Can you work these out from the model? Positions are in its coordinate system, mm. A direction names the side the tool comes from. Coordinates: 2 decimals unless noted, no trailing zeros. Loops run counter-clockwise (first coordinate to the right, second up) from the corner with the lowest first, then second, coordinate; pieces in that order, holes last.
```python
from build123d import *

# Parameters (mm, degrees)
SKETCH2_R           = 1.75
BOSS_EXTRUDE1_DEPTH = 5
FILLET1_R           = 5
SKETCH3_R           = 3.5
SKETCH3_W           = 2.1
SKETCH3_H           = 10.1
CUT_EXTRUDE1_DEPTH  = 6


with BuildPart() as part:
    # Sketch2 → Boss-Extrude1 (new body)
    with BuildSketch(Plane(origin=(0, 0, 0), x_dir=(1, 0, 0), z_dir=(0, 1, 0))):
        with BuildLine():
            Line((3, 28.141242251), (3, 32.361242251))
            ThreePointArc((3, 32.361242251), (0, 32.5), (-3, 32.361242251))
            Line((-3, 32.361242251), (-3, 28.141242251))
            Line((-3, 28.141242251), (-11.25, 28.141242251))
            Line((-11.25, 28.141242251), (-11.25, 22.141242251))
            Line((-11.25, 22.141242251), (-20.976543843, 22.141242251))
            ThreePointArc((-20.976543843, 22.141242251), (-30.5, 0), (-20.976543843, -22.141242251))
            Line((-20.976543843, -22.141242251), (-11.25, -22.141242251))
            Line((-11.25, -22.141242251), (-11.25, -28.141242251))
            Line((-11.25, -28.141242251), (-3, -28.141242251))
            Line((-3, -28.141242251), (-3, -32.361242251))
            ThreePointArc((-3, -32.361242251), (0, -32.5), (3, -32.361242251))
            Line((3, -32.361242251), (3, -28.141242251))
            Line((3, -28.141242251), (11.25, -28.141242251))
            Line((11.25, -28.141242251), (11.25, -22.141242251))
            Line((11.25, -22.141242251), (20.976543843, -22.141242251))
            ThreePointArc((20.976543843, -22.141242251), (30.5, 0), (20.976543843, 22.141242251))
            Line((20.976543843, 22.141242251), (11.25, 22.141242251))
            Line((11.25, 22.141242251), (11.25, 28.141242251))
            Line((11.25, 28.141242251), (3, 28.141242251))
        make_face()
        with Locations((0, 29.32)):
            Circle(SKETCH2_R, mode=Mode.SUBTRACT)
        with Locations((0, -29.32)):
            Circle(SKETCH2_R, mode=Mode.SUBTRACT)
    extrude(amount=BOSS_EXTRUDE1_DEPTH)

    # Fillet1
    fillet1_edges = [part.edges().sort_by_distance(p)[0] for p in [
        (-11.25, 2.5, -22.141242251),
        (11.25, 2.5, -22.141242251),
        (11.25, 2.5, 22.141242251),
        (-11.25, 2.5, 22.141242251),
    ]]
    fillet(fillet1_edges, radius=FILLET1_R)

    # Sketch3 → Cut-Extrude1 (cut, through all)
    with BuildSketch(Plane(origin=(0, 5, 0), x_dir=(1, 0, 0), z_dir=(0, 1, 0))):
        with Locations((10.253456157, 10.021242251)):
            Circle(SKETCH3_R)
        with Locations((-15.293456157, -16.411242251)):
            Circle(SKETCH3_R)
        with Locations((-20.976543843, -6.771242251)):
            Rectangle(SKETCH3_W, SKETCH3_H)
    extrude(amount=-CUT_EXTRUDE1_DEPTH, mode=Mode.SUBTRACT)


solid = part.part
```
Item 1: I need wall thicknesses on line 1 along Z through (x, y) = (0, 1.25); line 2 along Z through (x, y) = (-0.5, 1.1); line 3 along Z through (x, y) = (-5.5, 0.3). Which ranges of each line are inside material? Lowest first, please.
Results are:
line 1: z = -32.5 to -31.07, -27.57 to 27.57, 31.07 to 32.5
line 2: z = -32.5 to -31, -27.64 to 27.64, 31 to 32.5
line 3: z = -28.14 to 28.14
Item 2: Suppose I cut it at A-A, the plane z = 29.32. Please give me the cut outline in (x, y).
Results are:
outline: (-3, 0) - (-1.75, 0) - (-1.75, 5) - (-3, 5) - close; (1.75, 0) - (3, 0) - (3, 5) - (1.75, 5) - close
Item 3: Suppose I cut it at B-B, the plane x = 0. Please give me the cut outline in (y, z), plus the area to 3 significant figures.
Results are:
outline: (0, -32.5) - (5, -32.5) - (5, -31.07) - (0, -31.07) - close; (0, -27.57) - (5, -27.57) - (5, 27.57) - (0, 27.57) - close; (0, 31.07) - (5, 31.07) - (5, 32.5) - (0, 32.5) - close
area: 290 mm2
Item 4: We'd pull the mould along Z, two halves only. Please class faces 4 (the face through (-7, 2, 28.141)), 5 (the face through (-12.68, 2.54, -23.64)), 6 (the face through (13.592, 2.535, -11.073)): +Z half, -Z half, draft (parallel to the pull), parting line (faces both ways), or undercut.
Results are:
face 4: +Z half
face 5: -Z half
face 6: undercut
Item 5: Suppose I cut it at D-D, the plane z = 7. Please give me the cut outline in (x, y).
Results are:
outline: (-29.69, 0) - (-22.03, 0) - (-22.03, 5) - (-29.69, 5) - close; (-19.93, 0) - (29.69, 0) - (29.69, 5) - (-19.93, 5) - close
Item 6: I'm going to push flat-ended pins straight in: P1, Ø1.4, axis at x = 19, y = 2.5, coming from the +Z side; P2, Ø1.4, axis at x = -19, y = 3, coming from the -Z side; P3, Ø3, axis at x = -12, z = -16.5, coming from the -Y side; P4, Ø3, axis at x = 6.5, y = 4.5, coming from the +Z side. Where does each tip first touch, or does it pass through?
Results are:
P1: stops at z = 22.14
P2: stops at z = -22.14
P3: stops at y = 0
P4: stops at z = 28.14
Item 7: Suppose I cut it at C-C, the plane y = 3.45. Count the separate pieces of the cut face and the enclosed holes in it, plus the area to 3 significant figures.
Results are:
separate pieces: 1
enclosed holes: 5
area: 2,670 mm2
Item 8: On a 3-axis mill with a long thin cutter (end or side, diameter ignored), from which of +Z, -Z, +X, -X, +Y, -Y can I reach the whole of each face in a straight line? I mean faces 1 (the face through (-3, 2, -30)), 2 (the face through (3, 2, -30)), 3 (the face through (3, 2, 30)). Say none if no direction works.
Results are:
face 1: -Z, -X, +Y, -Y
face 2: -Z, +X, +Y, -Y
face 3: +Z, +X, +Y, -Y
